Autodesk Inventor part; units mm, degrees
ref_plane "YZ Plane" through (0, 0, 0) normal (1, 0, 0) x (0, 1, 0)
ref_plane "XZ Plane" through (0, 0, 0) normal (0, 1, 0) x (-1, 0, 0)
ref_plane "XY Plane" through (0, 0, 0) normal (0, 0, 1) x (1, 0, 0)
sketch "Sketch1" plane through (0, 0, 0) normal (0, 1, 0) x (-1, 0, 0)
  circle A0 centre (0, 0) radius 60
  dimension "d0" = 120
extrude "Extrusion1" add sketch "Sketch1" along normal mid plane 6.35
sketch "Sketch2" plane through (0, 3.175, 0) normal (0, 1, 0) x (1, 0, 0)
  circle A0 centre (0, 22.5) radius 2
  circle A1 centre (-15.9099, 15.9099) radius 2
  circle A2 centre (-22.5, 0) radius 2
  circle A3 centre (-15.9099, -15.9099) radius 2
  circle A4 centre (0, -22.5) radius 2
  circle A5 centre (15.9099, -15.9099) radius 2
  circle A6 centre (22.5, 0) radius 2
  circle A7 centre (15.9099, 15.9099) radius 2
  point P0 (0, 0)
  dimension "d3" = 4
  dimension "d4" = 22.5
  dimension "d7" = 360
extrude "Extrusion2" cut sketch "Sketch2" against normal through all
sketch "Sketch3" plane through (0, 3.175, 0) normal (0, 1, 0) x (1, 0, 0)
  circle A0 centre (-42, 20) radius 2.5 construction
  circle A1 centre (-48, 26) radius 2 construction
  circle A2 centre (-48, 14) radius 2 construction
  circle A3 centre (-36, 14) radius 2 construction
  circle A4 centre (-36, 26) radius 2 construction
  circle A5 centre (0, 0) radius 60 construction
  line L0 (0, 60) -> (0, -60) construction
  circle A6 centre (42, 20) radius 2.5 construction
  circle A7 centre (48, 26) radius 2 construction
  circle A8 centre (48, 14) radius 2 construction
  circle A9 centre (36, 14) radius 2 construction
  circle A10 centre (36, 26) radius 2 construction
  circle A11 centre (-20, -42) radius 2.5 construction
  circle A12 centre (-25, -37) radius 2 construction
  circle A13 centre (-25, -47) radius 2 construction
  circle A14 centre (-15, -47) radius 2 construction
  circle A15 centre (-15, -37) radius 2 construction
  circle A16 centre (20, -42) radius 2.5 construction
  circle A17 centre (25, -37) radius 2 construction
  circle A18 centre (25, -47) radius 2 construction
  circle A19 centre (15, -47) radius 2 construction
  circle A20 centre (15, -37) radius 2 construction
  circle A21 centre (-27.5, -42) radius 3
  line L1 (-60, 0) -> (60, 0) construction
  circle A22 centre (-16.5, -42) radius 3
  circle A23 centre (-5.5, -42) radius 3
  circle A24 centre (5.5, -42) radius 3
  circle A25 centre (16.5, -42) radius 3
  circle A26 centre (27.5, -42) radius 3
  line L2 (-5.5, -42) -> (5.5, -42) construction
  point P0 (0, -42)
  dimension "d11" = 5
  dimension "d12" = 42
  dimension "d13" = 20
  dimension "d14" = 4
  dimension "d15" = 6
  dimension "d16" = 6
  dimension "d19" = 360
  dimension "d23" = 5
  dimension "d24" = 42
  dimension "d25" = 20
  dimension "d26" = 4
  dimension "d27" = 5
  dimension "d28" = 5
  dimension "d31" = 360
  dimension "d49" = 6
  dimension "d52" = 11
extrude "Extrusion3" cut sketch "Sketch3" against normal through all
sketch "Sketch4" plane through (0, 3.175, 0) normal (0, 1, 0) x (1, 0, 0)
  circle A0 centre (-49, 42) radius 3 construction
  circle A1 centre (-49, 26) radius 4
  circle A2 centre (-49, 12) radius 4
  circle A3 centre (0, 0) radius 60 construction
  line L0 (-60, 0) -> (60, 0) construction
  circle A4 centre (-35, 42) radius 3
  circle A5 centre (-35, 26) radius 4
  circle A6 centre (-35, 12) radius 4
  line L1 (0, 60) -> (0, 0) construction
  circle A7 centre (49, 26) radius 4
  circle A8 centre (49, 12) radius 4
  circle A9 centre (35, 42) radius 3
  circle A10 centre (35, 26) radius 4
  circle A11 centre (35, 12) radius 4
  dimension "d33" = 6
  dimension "d34" = 8
  dimension "d35" = 8
  dimension "d36" = 16
  dimension "d37" = 14
  dimension "d40" = 14
  dimension "d45" = 35
  dimension "d46" = 12
extrude "Extrusion4" cut sketch "Sketch4" against normal through all
properties part number "TurretBasePlate"
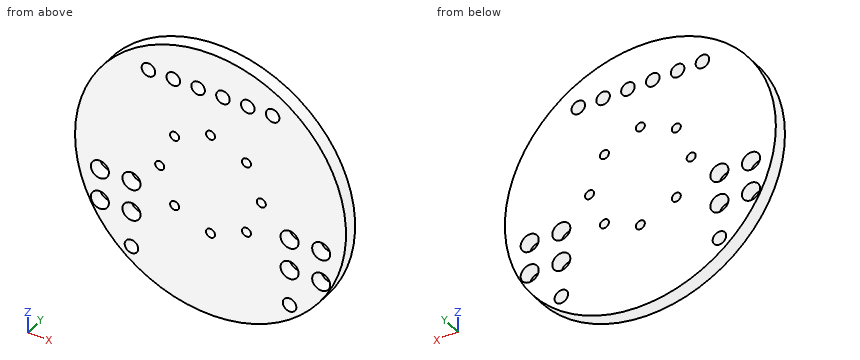
Part model, mm, in its own coordinate system. Round coordinates to 2 decimals unless told otherwise and drop trailing zeros. Loops run counter-clockwise (first coordinate to the right, second up) from the corner with the lowest first, then second, coordinate; pieces in that order, holes last.
Item 1: Cut at D-D, the plane z = -42. Give the cut face in (x, y) (3 decimals).
Item 2: Cut at B-B, the plane z = -12. Give the cut face in (x, y) (3 decimals), then the cut area to 3 significant figures.
Item 3: Drop flat-ended pins along their axis: P1, Ø3, axis at x = -21, y = 2.5, coming from the -Z side; P2, Ø3, axis at x = 0, z = 22.5, coming from the +Y side; P3, Ø2, axis at x = -0.5, y = -2, coming from the +Z side; P4, Ø1.5, axis at y = 2, z = -22, coming from the -X side. Give the stop position or say it passes through.
Item 4: Drill centre lines: line 1 (Z direction, x = -35, y = 1.5); line 2 (X direction, y = 3, z = -12); line 3 (X direction, y = -0.75, z = -22.5). Where is each one in solid material? Low to high.
Item 5: Cut at A-A, the plane x = -50. Give the cut face in (y, z) (3 decimals).
Item 6: Cut at C-C, the plane y = 1. State how many separate pieces and enclosed holes the cut face has, then the cut area to 3 significant figures.
A:
1. outline: (-42.849, -3.175) - (-38, -3.175) - (-38, 3.175) - (-42.849, 3.175) - close; (-32, -3.175) - (32, -3.175) - (32, 3.175) - (-32, 3.175) - close; (38, -3.175) - (42.849, -3.175) - (42.849, 3.175) - (38, 3.175) - close
2. outline: (-58.788, -3.175) - (-53, -3.175) - (-53, 3.175) - (-58.788, 3.175) - close; (-45, -3.175) - (-39, -3.175) - (-39, 3.175) - (-45, 3.175) - close; (-31, -3.175) - (31, -3.175) - (31, 3.175) - (-31, 3.175) - close; (39, -3.175) - (45, -3.175) - (45, 3.175) - (39, 3.175) - close; (53, -3.175) - (58.788, -3.175) - (58.788, 3.175) - (53, 3.175) - close
2. area: 543 mm2
3. P1: stops at z = -56.74
3. P2: passes through
3. P3: stops at z = 60
3. P4: stops at x = -56.11
4. line 1: z = -48.73 to -45, -39 to -30, -22 to -16, -8 to 48.73
4. line 2: x = -58.79 to -53, -45 to -39, -31 to 31, 39 to 45, 53 to 58.79
4. line 3: x = -55.62 to -50.94, -47.06 to -36.94, -33.06 to -2, 2 to 33.06, 36.94 to 47.06, 50.94 to 55.62
5. outline: (-3.175, -33.166) - (3.175, -33.166) - (3.175, -29.873) - (-3.175, -29.873) - close; (-3.175, -22.127) - (3.175, -22.127) - (3.175, -15.873) - (-3.175, -15.873) - close; (-3.175, -8.127) - (3.175, -8.127) - (3.175, 33.166) - (-3.175, 33.166) - close
6. separate pieces: 1
6. enclosed holes: 24
6. area: 10,600 mm2
